The model under review builds one solid part; all positions refer to its coordinate system, in mm. Face numbers are marked on the shaded views. A direction names the side the tool comes from. Coordinates: 2 decimals unless noted, no trailing zeros. Loops run counter-clockwise (first coordinate to the right, second up) from the corner with the lowest first, then second, coordinate; pieces in that order, holes last. Notation, with made-up numbers: M 51.5,-8.75 L 55.5,-8.75 A17 ccw 55.5,-1.75 Z; hole C -8.5,0 d10. An arc over 180 degrees is marked long. One line per item, written item: value.
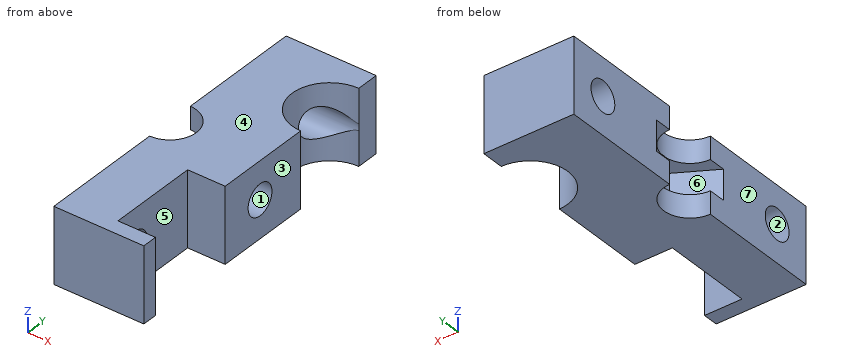
Autodesk Inventor part; units mm, degrees
ref_plane "Work Plane1" through (0, 0, 2.5) normal (0, 0, 1) x (1, 0, 0)
ref_plane "YZ Plane" through (0, 0, 0) normal (1, 0, 0) x (0, 1, 0)
ref_plane "XZ Plane" through (0, 0, 0) normal (0, 1, 0) x (-1, 0, 0)
sketch "Sketch1" plane through (0, 0, 0) normal (0, 0, 1) x (1, 0, 0)
  line L0 (10, -10) -> (-10, -10)
  line L1 (-10, -10) -> (-10, 10)
  line L2 (-10, 10) -> (10, 10)
  line L3 (10, 10) -> (10, -10)
  line L4 (10, -10) -> (-10, 10) construction
  line L5 (-10, -10) -> (10, 10) construction
  line L6 (10, -10) -> (6, -10)
  line L7 (6, -10) -> (6, 10)
  line L8 (6, 10) -> (10, 10)
  line L9 (10, 10) -> (10, -10)
  line L10 (6, 2) -> (4, 2)
  line L11 (4, 2) -> (4, -2)
  line L12 (4, -2) -> (6, -2)
  line L13 (6, -2) -> (6, 2)
  line L14 (0, 10) -> (0, -10)
  point P0 (0, 0)
  dimension "d0" = 20
  dimension "d1" = 20
  dimension "d2" = 4
  dimension "d6" = 2
  dimension "d7" = 2
  dimension "d8" = 4
  dimension "d9" = 2
  dimension "d44" = 6
extrude "Extrusion1" add sketch "Sketch1" along normal blind 5 contours L0 L14 L2 L7 L10 L11 L12
ref_plane "Work Plane1" through (0, 0, 2.5) normal (0, 0, 1) x (1, 0, 0)
sketch "Sketch2" plane through (0, 0, 2.5) normal (0, 0, 1) x (1, 0, 0)
  line L0 (0, 10) -> (0, -10)
  line L1 (0, 2.8868) -> (2.5, 1.4434)
  line L2 (2.5, 1.4434) -> (2.5, -1.4434)
  line L3 (2.5, -1.4434) -> (0, -2.8868)
  line L4 (0, -2.8868) -> (-2.5, -1.4434)
  line L5 (-2.5, -1.4434) -> (-2.5, 1.4434)
  line L6 (-2.5, 1.4434) -> (0, 2.8868)
  point P0 (0, 0)
  point P1 (0, 0)
  dimension "d12" = 5
extrude "Extrusion2" cut sketch "Sketch2" along normal mid plane 2
sketch "Sketch3" plane through (0, 0, 5) normal (0, 0, 1) x (1, 0, 0)
  circle A0 centre (0, 0) radius 1.75
  dimension "d15" = 3.5
extrude "Extrusion3" cut sketch "Sketch3" against normal blind 8
sketch "Sketch4" plane through (0, 10, 0) normal (-1, 0, 0) x (0, 0, 1)
  circle A0 centre (2.5, -2.5) radius 1.025
  circle A1 centre (2.5, -17.5) radius 1.025
  line L0 (0, 0) -> (5, 0)
  line L1 (0, 0) -> (0, -8.25)
  line L2 (0, -11.75) -> (0, -20)
  line L3 (0, -20) -> (5, -20)
  point P0 (0, -10)
  dimension "d18" = 2.05
  dimension "d19" = 2.05
  dimension "d20" = 2.5
  dimension "d21" = 2.5
  dimension "d22" = 2.5
  dimension "d23" = 2.5
extrude "Extrusion4" cut sketch "Sketch4" against normal blind 25
sketch "Sketch5" plane through (0, 0, 0) normal (0, 0, -1) x (-1, 0, 0)
  line L0 (-4, -2) -> (-4, 2)
  line L1 (-6, -10) -> (-6, -2)
  line L2 (-4, 2) -> (-6, 2)
  line L3 (-6, 2) -> (-6, -2)
  line L4 (-6, -2) -> (-4, -2)
  line L5 (-4, -2) -> (-4, 2)
  point P0 (0, 0)
extrude "Extrusion5" add sketch "Sketch5" against normal blind 5
sketch "Sketch6" plane through (0, 0, 0) normal (0, 0, -1) x (-1, 0, 0)
  line L0 (-6, -10) -> (-6, 10)
  circle A0 centre (-6, 6) radius 2.5
  line L1 (-6, -9) -> (-3.5, -9)
  line L2 (-3.5, -9) -> (-3.5, -3)
  line L3 (-3.5, -3) -> (-6, -3)
  line L4 (-6, -3) -> (-6, -9)
  line L5 (0, -10) -> (-6, -10)
  line L6 (-6, 10) -> (0, 10)
  point P0 (0, 0)
  point P1 (-6, 8.5)
  point P2 (-6, 3.5)
  dimension "d32" = 2.5
  dimension "d33" = 1
  dimension "d34" = 6
  dimension "d35" = 5
  dimension "d36" = 4
extrude "Extrusion6" cut sketch "Sketch6" against normal blind 5 contours L0 A0 | L0 L3 L2 L1 picked at (-5.3485, 6.5196)
sketch "Sketch7" plane through (6, -3, 0) normal (1, 0, 0) x (0, 0, -1)
  circle A0 centre (-2.5, 3) radius 1.025
  line L0 (-5, 0) -> (-5, 6.5)
  line L1 (0, -7) -> (-5, -7)
  point P0 (0, 3)
  dimension "d39" = 2.5
  dimension "d40" = 10
  dimension "d41" = 2.05
extrude "Extrusion7" cut sketch "Sketch7" against normal blind 12
equation "\"d18\" = d19"
properties part number "POMSliderMotor" material "Acetal Resin, White"
(1) Add section C-C on z = 2.5. State the section outline as (x, y) points (3 decimals), then the cut area to 3 significant figures.
Checks:
outline: M 0,-10 L 6,-10 L 6,-9 L 3.5,-9 L 3.5,-8.525 L 0,-8.525 Z; M 0,-6.475 L 3.5,-6.475 L 3.5,-3 L 6,-3 L 6,-1.025 L 2.5,-1.025 L 2.5,-1.443 L 0,-2.887 Z; M 0,2.887 L 2.5,1.443 L 2.5,1.025 L 6,1.025 L 6,3.5 A2.5 cw 3.546,6.475 L 0,6.475 Z; M 0,8.525 L 6,8.525 L 6,10 L 0,10 Z
area: 61.4 mm^2
(2) Tool access review of the marked faces 5, 6 and 7: name each direction out of +Z, -Z, +X, -X, +Y, -Y from which nothing blocks a thin tool from reaching the whole face with its end or side.
Checks:
face 5: +Z, -Z, +X
face 6: -X
face 7: +Z, -Z, -X, +Y, -Y
(3) To check wall thickness, follow L1, parallel to Y at x = 3.25, z = 2.5 (3 decimals); L2, parallel to Z at x = 3.85, y = 0 (3 decimals); L3, parallel to Y at x = 2.25, z = 3.4. State the ranges of each line that lie inside material, in increasing order. Write a range as [from, to].
Checks:
L1: [-10, -8.525], [-6.475, -1.025], [1.025, 6.475], [8.525, 10]
L2: [0, 1.475], [3.525, 5]
L3: [-10, -7.99], [-7.01, -1.59], [1.59, 7.01], [7.99, 10]
(4) Draft analysis for pull direction Z (two halves, no side actions). For the marked faces 1, 2, 3 and 4, state which applies: pulls with the +Z half, pulls with the -Z half, needs draft (parallel to the pull), parting line crosses it, or undercut.
Checks:
face 1: undercut
face 2: undercut
face 3: needs draft
face 4: pulls with the +Z half
(5) Add section A-A on y = -7.5. State the section outline as (x, z) points (3 decimals).
Checks:
outline: M 0,0 L 3.5,0 L 3.5,1.475 L 0,1.475 Z; M 0,3.525 L 3.5,3.525 L 3.5,5 L 0,5 Z
(6) Insertion check: pin 1 Ø1 at (y, z) = (1, 0.5) entering from -X; pin 2 Ø1.2 at (y, z) = (0, 2.5) entering from -X; pin 3 Ø0.8 at (x, y) = (0.5, -1.5) entering from -Z; pin 4 Ø2.5 at (y, z) = (-7.5, 2.5) entering from +X. Each pin has a flat end and moves straight along its axis. Give the tip position at first contact, or say it passes through.
Checks:
pin 1: x = 0.9
pin 2: through
pin 3: z = 0
pin 4: x = 3.5
(7) Add section B-B on x = 0.75. State the section outline as (y, z) points (3 decimals), then the cut area to 3 significant figures.
Checks:
outline: M -10,0 L -1.581,0 L -1.581,1.5 L -2.454,1.5 L -2.454,3.5 L -1.581,3.5 L -1.581,5 L -10,5 Z; M 1.581,0 L 10,0 L 10,5 L 1.581,5 L 1.581,3.5 L 2.454,3.5 L 2.454,1.5 L 1.581,1.5 Z; hole C -7.5,2.5 d2.05; hole C 7.5,2.5 d2.05
area: 74.1 mm^2
(8) Add section D-D on y = 0. State the section outline as (x, z) points (3 decimals).
Checks:
outline: M 1.75,0 L 6,0 L 6,1.475 L 1.75,1.475 Z; M 1.75,3.525 L 6,3.525 L 6,5 L 1.75,5 Z
